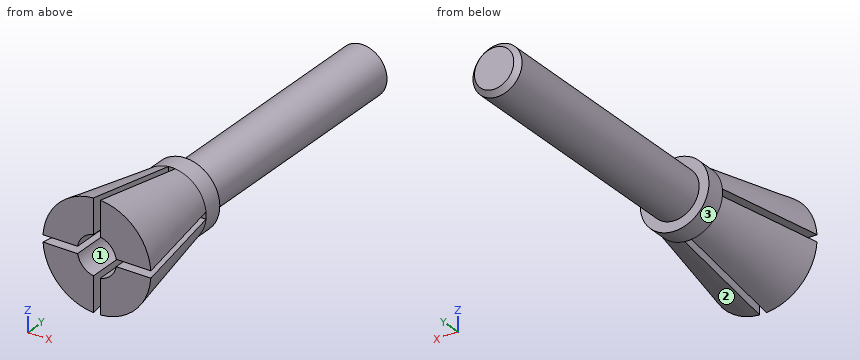
```python
from build123d import *

# Parameters (mm, degrees)
SKETCH1_R           = 5.5
BOSS_EXTRUDE1_DEPTH = 11
BOSS_EXTRUDE1_TAPER = 10.3
SKETCH2_R           = 3.500961199
BOSS_EXTRUDE2_DEPTH = 2
SKETCH3_R           = 2.5
BOSS_EXTRUDE3_DEPTH = 26.5
CHAMFER1_SIZE       = 0.5
CUT_EXTRUDE1_DEPTH  = 11


with BuildPart() as part:
    # Sketch1 → Boss-Extrude1 (new body)
    with BuildSketch(Plane(origin=(0, 0, 0), x_dir=(1, 0, 0), z_dir=(0, 1, 0))):
        Circle(SKETCH1_R)
    extrude(amount=BOSS_EXTRUDE1_DEPTH, taper=BOSS_EXTRUDE1_TAPER)

    # Sketch2 → Boss-Extrude2 (add)
    with BuildSketch(Plane(origin=(0, 11, 0), x_dir=(1, 0, 0), z_dir=(0, 1, 0))):
        with Locations(Location((0, 0, 0), (0, 0, 270))):
            Circle(SKETCH2_R)
    extrude(amount=BOSS_EXTRUDE2_DEPTH)

    # Sketch3 → Boss-Extrude3 (add)
    with BuildSketch(Plane(origin=(0, 13, 0), x_dir=(1, 0, 0), z_dir=(0, 1, 0))):
        with Locations(Location((0, 0, 0), (0, 0, 270))):
            Circle(SKETCH3_R)
    extrude(amount=BOSS_EXTRUDE3_DEPTH)

    # Chamfer1
    chamfer1_edges = [part.edges().sort_by_distance(p)[0] for p in [
        (0, 39.5, -2.5),
    ]]
    chamfer(chamfer1_edges, length=CHAMFER1_SIZE)

    # Sketch4 → Cut-Extrude1 (cut)
    with BuildSketch(Plane.XZ):
        with BuildLine():
            Line((0.35, 5.488852339), (0.35, 1.969136867))
            ThreePointArc((0.35, 1.969136867), (1.414213562, 1.414213562), (1.969136867, 0.35))
            Line((1.969136867, 0.35), (5.488852339, 0.35))
            ThreePointArc((5.488852339, 0.35), (5.5, 0), (5.488852339, -0.35))
            Line((5.488852339, -0.35), (1.969136867, -0.35))
            ThreePointArc((1.969136867, -0.35), (1.414213562, -1.414213562), (0.35, -1.969136867))
            Line((0.35, -1.969136867), (0.35, -5.488852339))
            ThreePointArc((0.35, -5.488852339), (0, -5.5), (-0.35, -5.488852339))
            Line((-0.35, -5.488852339), (-0.35, -1.969136867))
            ThreePointArc((-0.35, -1.969136867), (-1.414213562, -1.414213562), (-1.969136867, -0.35))
            Line((-1.969136867, -0.35), (-5.488852339, -0.35))
            ThreePointArc((-5.488852339, -0.35), (-5.5, 0), (-5.488852339, 0.35))
            Line((-5.488852339, 0.35), (-1.969136867, 0.35))
            ThreePointArc((-1.969136867, 0.35), (-1.414213562, 1.414213562), (-0.35, 1.969136867))
            Line((-0.35, 1.969136867), (-0.35, 5.488852339))
            ThreePointArc((-0.35, 5.488852339), (0, 5.5), (0.35, 5.488852339))
        make_face()
    extrude(amount=-CUT_EXTRUDE1_DEPTH, mode=Mode.SUBTRACT)


solid = part.part
```
Geometry: final body of the model. Coordinates: model frame, mm. Face numbers are marked on the shaded views. A direction names the side the tool comes from. Coordinates: 2 decimals unless noted, no trailing zeros. Order: outer loops, then holes, each group sorted by start corner. A loop starts at its lowest first (then second) coordinate and runs counter-clockwise, first axis right, second up. Notation, with made-up numbers: (67.25, -1.75) -> (118.25, -1.75) arc R15 cw to (118.25, 11.25) -> close; hole circle Ø9 at (82.25, 68). An arc over 180 degrees is marked (long way). Answer in a Markdown table with one row per item.
Item 1: Ray query, L1, parallel to Z at x = 0.5, y = 6.5; L2, parallel to X at y = 6, z = -2.5; L3, parallel to Y at x = 2.25, z = 2.5. Return the intervals inside material, ascending.
Return value:
| item | result |
|---|---|
| L1 | z = -4.29 to -1.94, 1.94 to 4.29 |
| L2 | x = -3.63 to -0.35, 0.35 to 3.63 |
| L3 | y = 0 to 13 |
Item 2: Section B-B on z = 0. Output: boundary loops of the cut face in (x, y).
Return value:
| item | result |
|---|---|
| outline | (-3.5, 11) -> (3.5, 11) -> (3.5, 13) -> (2.5, 13) -> (2.5, 39) -> (2, 39.5) -> (-2, 39.5) -> (-2.5, 39) -> (-2.5, 13) -> (-3.5, 13) -> close |
Item 3: Section C-C on y = 6. Output: boundary loops of the cut face in (x, z), plus the area to 3 significant figures.
Return value:
| item | result |
|---|---|
| outline | (-4.4, -0.35) arc R4.41 ccw to (-0.35, -4.4) -> (-0.35, -1.97) arc R2 cw to (-1.97, -0.35) -> close; (-4.4, 0.35) -> (-1.97, 0.35) arc R2 cw to (-0.35, 1.97) -> (-0.35, 4.4) arc R4.41 ccw to start; (0.35, -4.4) arc R4.41 ccw to (4.4, -0.35) -> (1.97, -0.35) arc R2 cw to (0.35, -1.97) -> close; (0.35, 1.97) arc R2 cw to (1.97, 0.35) -> (4.4, 0.35) arc R4.41 ccw to (0.35, 4.4) -> close |
| area | 41.8 mm² |
Item 4: Section D-D on y = 30. Output: boundary loops of the cut face in (x, z).
Return value:
| item | result |
|---|---|
| outline | circle Ø5 at (0, 0) |
Item 5: Contact query for flat-ended pins moving along their axis: P1, Ø4, axis at x = 2.5, z = 4, coming from the +Y side; P2, Ø1.8, axis at y = 6.5, z = -4.5, coming from the +X side; P3, Ø1, axis at x = -4, z = -0.5, coming from the -Y side; P4, Ø1.8, axis at x = 3.5, y = 6.5, coming from the +Z side. Output: stop coordinate, or through.
Return value:
| item | result |
|---|---|
| P1 | stops at y = 13 |
| P2 | stops at x = 2.42 |
| P3 | stops at y = 0 |
| P4 | stops at z = 3.48 |
Item 6: Section A-A on x = 0. Output: boundary loops of the cut face in (y, z), plus the area to 3 significant figures.
Return value:
| item | result |
|---|---|
| outline | (11, -3.5) -> (13, -3.5) -> (13, -2.5) -> (39, -2.5) -> (39.5, -2) -> (39.5, 2) -> (39, 2.5) -> (13, 2.5) -> (13, 3.5) -> (11, 3.5) -> close |
| area | 146 mm² |
Item 7: Access query for the marked faces 1, 2 and 3. Directions: +Z, -Z, +X, -X, +Y, -Y. A direction counts if a zero-diameter tool reaches every point of the face in a straight line with its end or side. Return the directions, or none.
Return value:
| item | result |
|---|---|
| face 1 | -Y |
| face 2 | -Z, +X, +Y |
| face 3 | +Y |
